For this review, take the finished solid that the model builds, in its own axes (mm). Face numbers are marked on the shaded views. A direction names the side the tool comes from. Coordinates: 2 decimals unless noted, no trailing zeros. Loops run counter-clockwise (first coordinate to the right, second up) from the corner with the lowest first, then second, coordinate; pieces in that order, holes last. Notation, with made-up numbers: (69.25, -5.5) -> (80.25, -5.5) arc R29 ccw to (80.25, 31.5) -> close; hole circle Ø7 at (72, 66). An arc over 180 degrees is marked (long way). Answer in a Markdown table with one row per item.
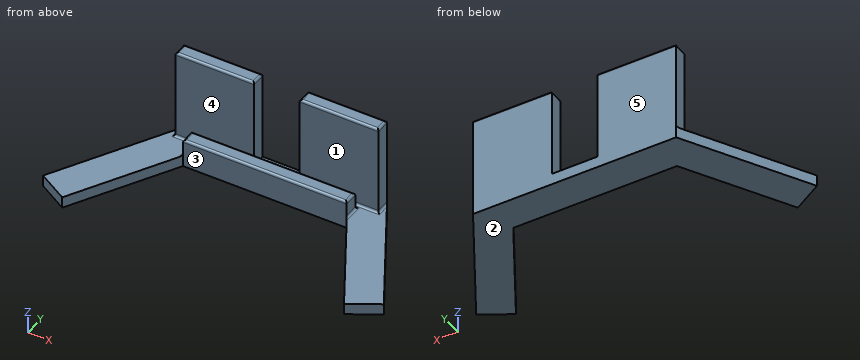
from build123d import *

# Parameters (mm, degrees)
F1_DEPTH = 6.35
F2_W     = 44.055171
F2_H     = 7.9375
F3_DEPTH = 50.8
F4_W     = 91.513296
F4_H     = 7.9375
F5_DEPTH = 9.525
F6_R     = 1.27


with BuildPart() as f1:
    # F0 (on Top) → F1 (new body)
    with BuildSketch(Plane.XY):
        Polygon((56.755171, 0), (-56.755171, 0), (-95.25, -66.675), (-78.752216, -76.2), (-45.756648, -19.05), (0, -19.05), (45.756648, -19.05), (78.752216, -76.2), (95.25, -66.675), align=None)
    extrude(amount=F1_DEPTH)

    # F2 (on face) → F3 (join)
    with BuildSketch(Plane.XY.offset(6.35)):
        with Locations((-34.727585, -3.96875)):
            Rectangle(F2_W, F2_H)
        with Locations((34.727585, -3.96875)):
            Rectangle(F2_W, F2_H)
    extrude(amount=F3_DEPTH)

    # F4 (on face) → F5 (join)
    with BuildSketch(Plane.XY.offset(6.35)):
        with Locations((0, -15.08125)):
            Rectangle(F4_W, F4_H)
    extrude(amount=F5_DEPTH)

    # F6
    f6_edges = [f1.edges().sort_by_distance(p)[0] for p in [
        (-45.756648, -15.08125, 15.875),
        (0, -19.05, 15.875),
        (45.756648, -15.08125, 15.875),
        (0, -11.1125, 15.875),
        (-34.727585, 0, 57.15),
        (-56.755171, -3.96875, 57.15),
        (-34.727585, -7.9375, 57.15),
        (-12.7, -3.96875, 57.15),
        (34.727585, -7.9375, 57.15),
        (56.755171, -3.96875, 57.15),
        (34.727585, 0, 57.15),
        (12.7, -3.96875, 57.15),
        (-56.755171, -3.96875, 6.35),
        (-34.727585, -7.9375, 6.35),
        (-45.756648, -15.08125, 6.35),
        (0, -11.1125, 6.35),
        (34.727585, -7.9375, 6.35),
        (45.756648, -15.08125, 6.35),
        (56.755171, -3.96875, 6.35),
    ]]
    fillet(f6_edges, radius=F6_R)


solid = f1.part
Item 1: The part is to be moulded in two halves that separate along Y. For the marked faces 1, 2 and 3, say which applies: +Y half, -Y half, draft (parallel to the pull), parting line (faces both ways), or undercut.
Worked answers:
| item | result |
|---|---|
| face 1 | undercut |
| face 2 | draft |
| face 3 | -Y half |
Item 2: For the marked faces 4 and 5, list the 3-axis set-ups (+Z, -Z, +X, -X, +Y, -Y) from which the entire face can be reached by the end or side of a thin tool; tool diameter is ignored.
Worked answers:
| item | result |
|---|---|
| face 4 | +Z, +X, -X |
| face 5 | +Z, -Z, +X, -X, +Y |
Item 3: Insertion check: pin 1 (10 mm diameter, centred on y = -20.5, z = 6, fed in from -X); pin 2 (5 mm diameter, centred on x = 51, y = -33, fed in from +Z); pin 3 (2 mm diameter, centred on x = 10, z = 12.5, fed in from +Y). Each pin has a flat end and moves straight along its axis. Give the tip position at first contact, or say it passes through.
Worked answers:
| item | result |
|---|---|
| pin 1 | x = -71.48 |
| pin 2 | z = 6.35 |
| pin 3 | y = -11.11 |
Item 4: For L1, parallel to X at y = -4, z = 32.5; L2, parallel to Y at x = 52.5, z = 11.5; L3, parallel to X at y = -17, z = 10.5, list the stretches that pass through material, from the lowest coordinate up.
Worked answers:
| item | result |
|---|---|
| L1 | -56.76 to -12.7, 12.7 to 56.76 |
| L2 | -7.94 to 0 |
| L3 | -45.76 to 45.76 |
Item 5: Take a section at A-A, the plane z = 48. State the section outline as (x, y) points, and give its area (3 significant figures).
Worked answers:
| item | result |
|---|---|
| outline | (-56.76, -7.94) -> (-12.7, -7.94) -> (-12.7, 0) -> (-56.76, 0) -> close; (12.7, -7.94) -> (56.76, -7.94) -> (56.76, 0) -> (12.7, 0) -> close |
| area | 699 mm² |
Item 6: Take a section at C-C, the plane y = -38. State the section outline as (x, z) points, and give its area (3 significant figures).
Worked answers:
| item | result |
|---|---|
| outline | (-78.69, 0) -> (-56.7, 0) -> (-56.7, 6.35) -> (-78.69, 6.35) -> close; (56.7, 0) -> (78.69, 0) -> (78.69, 6.35) -> (56.7, 6.35) -> close |
| area | 279 mm² |
